Autodesk Inventor part; units mm, degrees
ref_plane "YZ Plane" through (0, 0, 0) normal (1, 0, 0) x (0, 1, 0)
ref_plane "XZ Plane" through (0, 0, 0) normal (0, 1, 0) x (-1, 0, 0)
ref_plane "XY Plane" through (0, 0, 0) normal (0, 0, 1) x (1, 0, 0)
sketch "Sketch1" plane through (0, 0, 0) normal (0, 1, 0) x (-1, 0, 0)
  circle A0 centre (0, 0) radius 12.75
  circle A1 centre (0, 0) radius 30
  dimension "d0" = 25.5
  dimension "d1" = 60
extrude "Extrusion1" add sketch "Sketch1" along normal blind 7
sketch "Sketch2" plane through (0, 7, 0) normal (0, 1, 0) x (1, 0, 0)
  circle A0 centre (0, 0) radius 30
extrude "Extrusion2" add sketch "Sketch2" along normal blind 3
sketch "Sketch3" plane through (0, 0, 0) normal (0, -1, 0) x (1, 0, 0)
  circle A0 centre (0, 0) radius 30
  line L0 (0, 30) -> (0, 25)
  point P0 (-21.6506, 12.5)
  point P1 (-21.6506, -12.5)
  point P2 (0, -25)
  point P3 (21.6506, -12.5)
  point P4 (21.6506, 12.5)
  dimension "d6" = 5
  dimension "d9" = 360
hole "Hole1" at (0, 0, 25) at (-21.6506, 0, 12.5) at (-21.6506, 0, -12.5) at (0, 0, -25) at (21.6506, 0, -12.5) at (21.6506, 0, 12.5) direction (0, 1, 0) diameter 3 end through all countersink diameter 5.5 countersink angle 90
properties part number "Base_To_First_Tilt_Attachment"
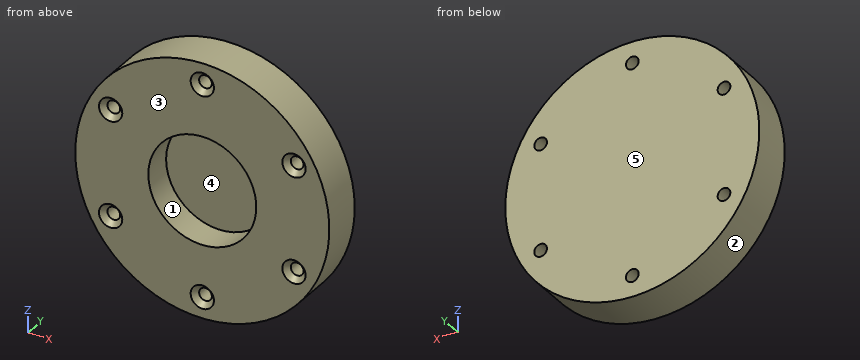
Here's how the part is built. I have some questions about the finished solid (model axes, mm). Face numbers are marked on the shaded views. A direction names the side the tool comes from. Round coordinates to 2 decimals unless told otherwise and drop trailing zeros. Write each loop counter-clockwise with the first axis right and the second up, starting at its lowest first coordinate (ties: lowest second). Pieces come first, ordered by that corner, then holes. Notation, with made-up numbers: (-13, 79) -> (45, 79) arc R23 ccw to (45, 87) -> close; hole circle Ø10 at (7, 15.25). An arc over 180 degrees is marked (long way). One line per item, written item: value.
1) Suppose I cut it at D-D on z = -2.5. List the corners of the cut face in (x, y) for me.
Filled sheet:
outline: (-29.9, 0) -> (-12.5, 0) -> (-12.5, 7) -> (12.5, 7) -> (12.5, 0) -> (29.9, 0) -> (29.9, 10) -> (-29.9, 10) -> close
2) I'm going to push flat-ended pins straight in: pin 1 Ø2.5 at (x, z) = (-21.65, -12.5) entering from +Y; pin 2 Ø4 at (x, z) = (0, -25) entering from -Y; pin 3 Ø1.5 at (x, y) = (22, 4) entering from -Z; pin 4 Ø1.5 at (x, y) = (24, 9) entering from -Z. Where does each tip first touch, or does it pass through?
Filled sheet:
pin 1: passes through
pin 2: stops at y = 0.75
pin 3: stops at z = -21.18
pin 4: stops at z = -18.96
3) Suppose I cut it at B-B on y = 9. List the corners of the cut face in (x, z) for me, plus the area to 3 significant figures.
Filled sheet:
outline: circle Ø60 at (0, 0); hole circle Ø3 at (-21.65, -12.5); hole circle Ø3 at (-21.65, 12.5); hole circle Ø3 at (0, -25); hole circle Ø3 at (0, 25); hole circle Ø3 at (21.65, -12.5); hole circle Ø3 at (21.65, 12.5)
area: 2,790 mm2
4) Suppose I cut it at C-C on y = 3.5. List the corners of the cut face in (x, z) for me, plus the area to 3 significant figures.
Filled sheet:
outline: circle Ø60 at (0, 0); hole circle Ø3 at (-21.65, -12.5); hole circle Ø3 at (-21.65, 12.5); hole circle Ø25.5 at (0, 0); hole circle Ø3 at (0, -25); hole circle Ø3 at (0, 25); hole circle Ø3 at (21.65, -12.5); hole circle Ø3 at (21.65, 12.5)
area: 2,270 mm2
5) If I drill on line 1 (Z direction, x = 0, y = 5.5); line 2 (X direction, y = 7.25, z = -12.5); line 3 (Z direction, x = 0, y = 8), over which ranges is the centre line in solid material (lowest first)? Write a range as [from, to].
Filled sheet:
line 1: z = [-30, -26.5], [-23.5, -12.75], [12.75, 23.5], [26.5, 30]
line 2: x = [-27.27, -23.15], [-20.15, 20.15], [23.15, 27.27]
line 3: z = [-30, -26.5], [-23.5, 23.5], [26.5, 30]
6) We'd pull the mould along Z, two halves only. Please class the marked faces 1, 2 and 3: released by +Z, released by -Z, zero draft, split by the parting line, or undercut.
Filled sheet:
face 1: undercut
face 2: split by the parting line
face 3: zero draft
7) For the marked faces 4 and 5, which set-ups out of +Z, -Z, +X, -X, +Y, -Y let a thin tool reach every point of the face, with its end or its side?
Filled sheet:
face 4: -Y
face 5: +Z, -Z, +X, -X, +Y
